Geometry: final body of the model. Coordinates: model frame, mm. Face numbers are marked on the shaded views. Coordinates: 2 decimals unless noted, no trailing zeros. Order: outer loops, then holes, each group sorted by start corner. A loop starts at its lowest first (then second) coordinate and runs counter-clockwise, first axis right, second up. Notation, with made-up numbers: (82, -18) -> (129, -18) arc R20 cw to (129, 6) -> close; hole circle Ø10 at (44, 66). An arc over 180 degrees is marked (long way). Use one line per item in the form item = value.
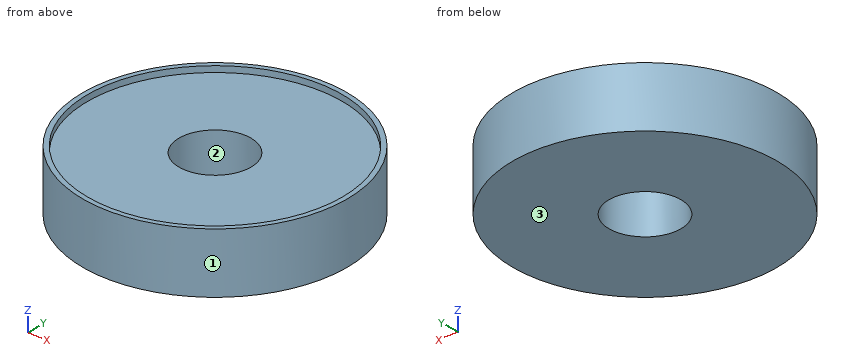
```python
from build123d import *

# Parameters (mm, degrees)
CYLINDER036_R     = 10.6
CYLINDER036_DEPTH = 10
CYLINDER034_R     = 3
CYLINDER034_DEPTH = 5
CYLINDER035_R     = 11
CYLINDER035_DEPTH = 5


with BuildPart() as cylinder036:
    # Cylinder036 → Cylinder036 (new body)
    with BuildSketch(Plane.XY.offset(4.5)):
        Circle(CYLINDER036_R)
    extrude(amount=CYLINDER036_DEPTH)


with BuildPart() as cylinder034:
    # Cylinder034 → Cylinder034 (new body)
    with BuildSketch(Plane.XY):
        Circle(CYLINDER034_R)
    extrude(amount=CYLINDER034_DEPTH)


with BuildPart() as cut030:
    # Cylinder035 → Cylinder035 (new body)
    with BuildSketch(Plane.XY):
        Circle(CYLINDER035_R)
    extrude(amount=CYLINDER035_DEPTH)

    # Cut029: cut Cylinder034
    add(cylinder034.part, mode=Mode.SUBTRACT)

    # Cut030: cut Cylinder036
    add(cylinder036.part, mode=Mode.SUBTRACT)


solid = cut030.part
```
1) Pull-direction query (X, two-part tool) for the marked faces 1, 2 and 3; classes: released by +X, released by -X, zero draft, split by the parting line, or undercut.
Results found:
face_1 = split by the parting line
face_2 = undercut
face_3 = zero draft
2) Section D-D, the plane x = -4. Output: boundary loops of the cut face in (y, z).
Results found:
outline = (-10.25, 0) -> (10.25, 0) -> (10.25, 5) -> (9.82, 5) -> (9.82, 4.5) -> (-9.82, 4.5) -> (-9.82, 5) -> (-10.25, 5) -> close
3) Contact query for flat-ended pins moving along their axis: P1, Ø3, axis at y = -5.5, z = 0.5, coming from the -X side; P2, Ø5, axis at x = -4.5, y = -7, coming from the -Z side; P3, Ø1.5, axis at x = -6, z = 0.5, coming from the -Y side; P4, Ø1, axis at y = -7.5, z = 1, coming from the -X side. Output: stop coordinate, or through.
Results found:
P1 = -10.25
P2 = 0
P3 = -9.67
P4 = -8.49
4) Section C-C, the plane z = 2.85. Output: boundary loops of the cut face in (x, y), and give its area (3 significant figures).
Results found:
outline = circle Ø22 at (0, 0); hole circle Ø6 at (0, 0)
area = 352 mm2
5) Section A-A, the plane x = 0. Output: boundary loops of the cut face in (y, z).
Results found:
outline = (-11, 0) -> (-3, 0) -> (-3, 4.5) -> (-10.6, 4.5) -> (-10.6, 5) -> (-11, 5) -> close; (3, 0) -> (11, 0) -> (11, 5) -> (10.6, 5) -> (10.6, 4.5) -> (3, 4.5) -> close
6) Material intervals for probe 1 along Y at (x, z) = (0, 2.6); probe 2 along Y at (x, z) = (0, 4.8); probe 3 along Z at (x, y) = (5.75, -4), sorted ascending. Write a range as from..to.
Results found:
probe_1 = -11..-3, 3..11
probe_2 = -11..-10.6, 10.6..11
probe_3 = 0..4.5
